```python
from build123d import *

# Parameters (mm, degrees)
SKETCH_W        = 24
SKETCH_H        = 10
PAD_DEPTH       = 15.8
SKETCH001_R     = 0.2
SKETCH001_W     = 0.8
SKETCH001_H     = 0.2
PAD001_DEPTH    = 2
FILLET_R        = 1
FILLET001_R     = 1
FILLET002_R     = 1
FILLET003_R     = 1
CHAMFER_SIZE    = 0.1
CHAMFER001_SIZE = 0.1
CHAMFER002_SIZE = 0.1
CHAMFER003_SIZE = 0.1
FILLET004_R     = 0.1


with BuildPart() as part:
    # Sketch → Pad (new body)
    with BuildSketch(Plane.XY):
        with Locations((12, -5)):
            Rectangle(SKETCH_W, SKETCH_H)
    extrude(amount=PAD_DEPTH)

    # Sketch001 → Pad001 (join)
    with BuildSketch(Plane.XY):
        with Locations((1.5, -1.25)):
            Circle(SKETCH001_R)
        with Locations((1.5, -8.75)):
            Circle(SKETCH001_R)
        with Locations((18.7, -1.25)):
            Rectangle(SKETCH001_W, SKETCH001_H)
        with Locations((22.2, -8.75)):
            Rectangle(SKETCH001_W, SKETCH001_H)
    extrude(amount=-PAD001_DEPTH)

    # Fillet
    fillet_edges = [part.edges().sort_by_distance(p)[0] for p in [
        (12, -10, 15.8),
    ]]
    fillet(fillet_edges, radius=FILLET_R)

    # Fillet001
    fillet001_edges = [part.edges().sort_by_distance(p)[0] for p in [
        (24, -4.5, 15.8),
    ]]
    fillet(fillet001_edges, radius=FILLET001_R)

    # Fillet002
    fillet002_edges = [part.edges().sort_by_distance(p)[0] for p in [
        (11.5, 0, 15.8),
    ]]
    fillet(fillet002_edges, radius=FILLET002_R)

    # Fillet003
    fillet003_edges = [part.edges().sort_by_distance(p)[0] for p in [
        (0, -5, 15.8),
    ]]
    fillet(fillet003_edges, radius=FILLET003_R)

    # Chamfer
    chamfer_edges = [part.edges().sort_by_distance(p)[0] for p in [
        (19.1, -1.25, -2),
    ]]
    chamfer(chamfer_edges, length=CHAMFER_SIZE)

    # Chamfer001
    chamfer001_edges = [part.edges().sort_by_distance(p)[0] for p in [
        (18.3, -1.25, -2),
    ]]
    chamfer(chamfer001_edges, length=CHAMFER001_SIZE)

    # Chamfer002
    chamfer002_edges = [part.edges().sort_by_distance(p)[0] for p in [
        (21.8, -8.75, -2),
    ]]
    chamfer(chamfer002_edges, length=CHAMFER002_SIZE)

    # Chamfer003
    chamfer003_edges = [part.edges().sort_by_distance(p)[0] for p in [
        (22.6, -8.75, -2),
    ]]
    chamfer(chamfer003_edges, length=CHAMFER003_SIZE)

    # Fillet004
    fillet004_edges = [part.edges().sort_by_distance(p)[0] for p in [
        (1.3, -8.75, -2),
        (1.3, -1.25, -2),
    ]]
    fillet(fillet004_edges, radius=FILLET004_R)


solid = part.part
```
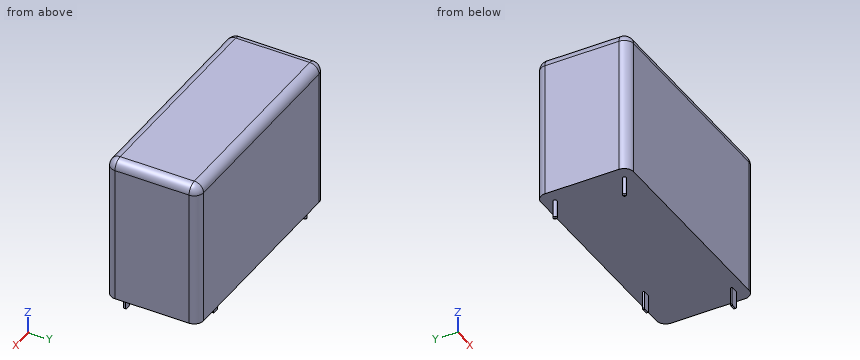
Read the model definition and answer for the solid it produces. Units are mm, in the model's axes. Give positions to 0.01 mm unless a question says otherwise; leave off trailing zeros. Order: outer loops, then holes, each group sorted by start corner. A loop starts at its lowest first (then second) coordinate and runs counter-clockwise, first axis right, second up. Notation, with made-up numbers: (41.5, 64) -> (81.5, 64) arc R25 ccw to (81.5, 80) -> close; hole circle Ø10 at (16, 21.25). An arc over 180 degrees is marked (long way). Write item = value, one per line.
1. Straight lines are drawn through the part: line 1 along Z through (x, y) = (4.75, -4.75); line 2 along X through (y, z) = (-9.5, 7.5). For each, find the intervals that lie inside material, in ascending order.
Numbers:
line_1 = 0 to 15.8
line_2 = 0.13 to 23.87
2. A cutting plane is placed at A-A, the plane y = -3.25. Write down the section's boundary in (x, z).
Numbers:
outline = (0, 0) -> (24, 0) -> (24, 14.8) arc R1 ccw to (23, 15.8) -> (1, 15.8) arc R1 ccw to (0, 14.8) -> close
3. A cutting plane is placed at B-B, the plane x = 13. Write down the section's boundary in (y, z), and give its area (3 significant figures).
Numbers:
outline = (-10, 0) -> (0, 0) -> (0, 14.8) arc R1 ccw to (-1, 15.8) -> (-9, 15.8) arc R1 ccw to (-10, 14.8) -> close
area = 158 mm²
4. Given pin 1 (0.9 mm diameter, centred on x = 18.5, z = -0.5, fed in from -Y); pin 2 (0.9 mm diameter, centred on x = 22.5, z = -1.5, fed in from -Y); pin 3 (0.6 mm diameter, centred on x = 22.5, z = -0.5, fed in from +Y), each flat-ended and moving along its own axis, determine where each tip first touches the part or whether it passes through.
Numbers:
pin_1 = -1.35
pin_2 = -8.85
pin_3 = -8.65
